Check sheet for the drawn part. Datum: minimum x, y, z corner. Units: mm. Give positions to 0.01 mm unless a question says otherwise; leave off trailing zeros. Write each loop counter-clockwise with the first axis right and the second up, starting at its lowest first coordinate (ties: lowest second). Pieces come first, ordered by that corner, then holes.
(1) Cross-section at D-D (z = 29.5). Record the boundary of the cut face in (x, y).
(2) Depth check by flat-ended pin: P1, Ø7, axis at x = 15, z = 55, coming from the +Y side; P2, Ø1, axis at x = 33, y = 5.5, coming from the -Z side; P3, Ø1, axis at x = 21.5, y = 1.5, coming from the +Z side. Enter the tip coordinate at first touch or a pass-through.
(3) Cross-section at C-C (x = 35). Record the boundary of the cut face in (y, z).
(4) Cross-section at B-B (z = 55). Record the boundary of the cut face in (x, y), and give its area (3 significant figures).
(5) Thickness scan on line 1 along Z through (x, y) = (15, 0.4); line 2 along X through (y, z) = (0.5, 17.5); line 3 along Z through (x, y) = (53.5, 1.75). Record the ranges inside material, lowest first.
(6) Cross-section at A-A (x = 15). Record the boundary of the cut face in (y, z).
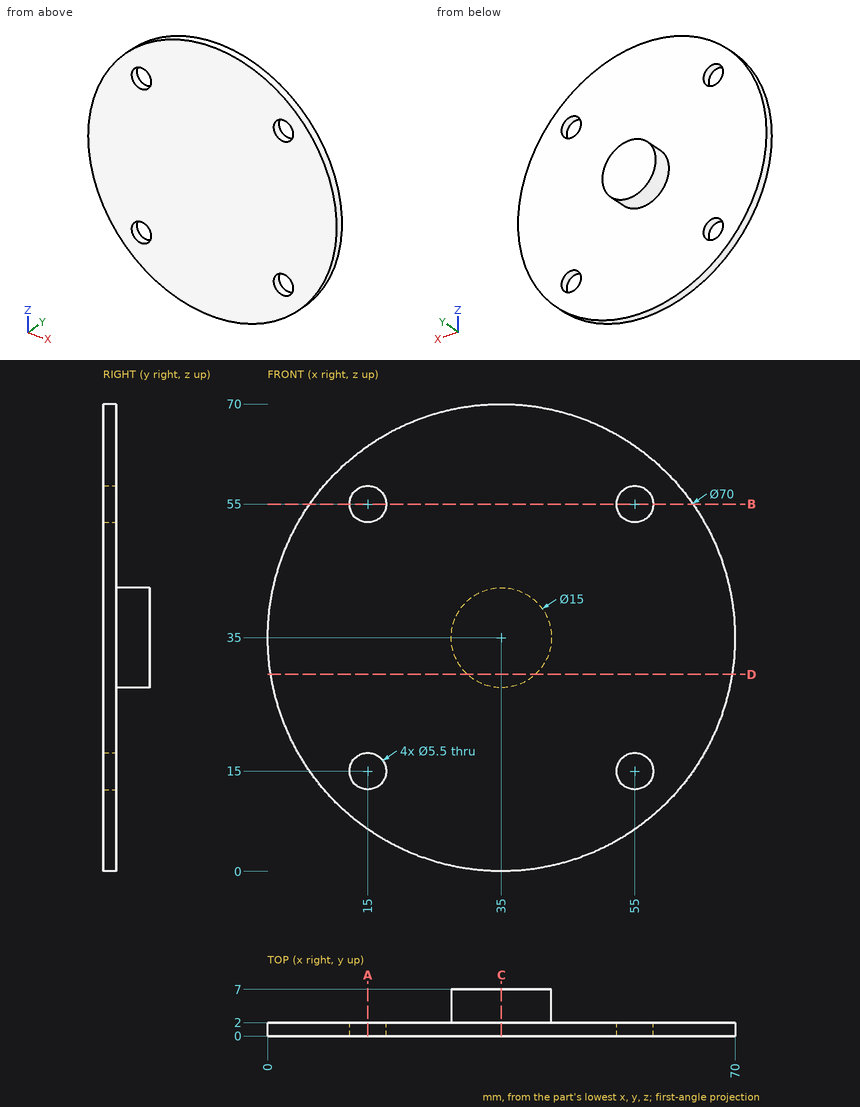
Reply:
1. outline: (0.43, 0) - (69.57, 0) - (69.57, 2) - (40.1, 2) - (40.1, 7) - (29.9, 7) - (29.9, 2) - (0.43, 2) - close
2. P1: stops at y = 2
2. P2: stops at z = 27.65
2. P3: stops at z = 67.5
3. outline: (0, 0) - (2, 0) - (2, 27.5) - (7, 27.5) - (7, 42.5) - (2, 42.5) - (2, 70) - (0, 70) - close
4. outline: (6.28, 0) - (12.25, 0) - (12.25, 2) - (6.28, 2) - close; (17.75, 0) - (52.25, 0) - (52.25, 2) - (17.75, 2) - close; (57.75, 0) - (63.72, 0) - (63.72, 2) - (57.75, 2) - close
4. area: 92.9 mm2
5. line 1: z = 6.28 to 12.25, 17.75 to 52.25, 57.75 to 63.72
5. line 2: x = 4.69 to 13.85, 16.15 to 53.85, 56.15 to 65.31
5. line 3: z = 5.29 to 12.7, 17.3 to 52.7, 57.3 to 64.71
6. outline: (0, 6.28) - (2, 6.28) - (2, 12.25) - (0, 12.25) - close; (0, 17.75) - (2, 17.75) - (2, 52.25) - (0, 52.25) - close; (0, 57.75) - (2, 57.75) - (2, 63.72) - (0, 63.72) - close
